Autodesk Inventor part; units mm, degrees
ref_plane "YZ Plane" through (0, 0, 0) normal (1, 0, 0) x (0, 1, 0)
ref_plane "XZ Plane" through (0, 0, 0) normal (0, 1, 0) x (-1, 0, 0)
ref_plane "XY Plane" through (0, 0, 0) normal (0, 0, 1) x (1, 0, 0)
sketch "スケッチ1" plane through (0, 0, 0) normal (0, 0, 1) x (1, 0, 0)
  line L0 (-40, 18) -> (40, 18)
  line L1 (40, 18) -> (40, -18)
  line L2 (40, -18) -> (-40, -18)
  line L3 (-40, -18) -> (-40, 18)
  line L4 (0, 0) -> (0, 18) construction
  line L5 (0, 0) -> (40, 0) construction
  dimension "d0" = 36
  dimension "d1" = 80
extrude "プレート1" add sketch "スケッチ1" along normal blind 5
sketch "スケッチ2" plane through (0, 0, 5) normal (0, 0, 1) x (1, 0, 0)
  line L0 (40, 18) -> (40, -18)
  line L1 (-40, 18) -> (-40, -18)
  line L2 (-40, 0) -> (40, 0) construction
  point P0 (22, 0)
  point P1 (11.8, 0)
  point P2 (27.1, -8.8335)
  point P3 (27.1, 8.8335)
  dimension "d3" = 10.2
  dimension "d6" = 360
  dimension "d116" = 18
hole "穴1" at (11.8, 0, 5) at (27.1, -8.8335, 5) at (27.1, 8.8335, 5) direction (0, 0, -1) diameter 4 depth 5
sketch "スケッチ3" plane through (0, 0, 5) normal (0, 0, 1) x (1, 0, 0)
  line L0 (40, 18) -> (40, -18)
  point P0 (22, 0)
  point P1 (22, -12.5)
  point P2 (32.8253, -6.25)
  point P3 (32.8253, 6.25)
  point P4 (22, 12.5)
  point P5 (11.1747, 6.25)
  point P6 (11.1747, -6.25)
  dimension "d15" = 12.5
  dimension "d18" = 360
  dimension "d117" = 18
hole "穴2" at (22, -12.5, 5) at (32.8253, -6.25, 5) at (32.8253, 6.25, 5) at (22, 12.5, 5) at (11.1747, 6.25, 5) at (11.1747, -6.25, 5) direction (0, 0, -1) diameter 3.2 depth 5
sketch "スケッチ13" plane through (0, 0, 0) normal (0, 0, -1) x (-1, 0, 0)
  line L0 (0, 0) -> (40, 0) construction
  line L1 (40, -18) -> (40, 18)
  line L2 (-40, 18) -> (-40, -18)
  point P0 (33, 0)
  point P1 (3, 0)
  dimension "d127" = 30
  dimension "d128" = 43
hole "穴10" at (-33, 0, 0) at (-3, 0, 0) direction (0, 0, 1) diameter 7.9 depth 5
fillet "フィレット1" radius 10 4 edges at (40, -18, 2.5) (40, 18, 2.5) (-40, 18, 2.5) (-40, -18, 2.5)
equation "\"d13\" = d3"
equation "\"d125\" = Thickness"
equation "\"d2\" = Thickness"
equation "\"BendRadius\" = Thickness"
equation "\"BendReliefWidth\" = Thickness"
equation "\"BendReliefDepth\" = 0.5 * Thickness"
equation "\"TransitionRadius\" = BendRadius"
equation "\"JacobiRadiusSize\" = BendRadius"
equation "\"GapSize\" = Thickness"
properties part number "link_plate" material "アルミニウム 6061"
CAD build for the part. Positions are in the model's coordinates, mm. Round coordinates to 2 decimals unless told otherwise and drop trailing zeros. Loops run counter-clockwise (first coordinate to the right, second up) from the corner with the lowest first, then second, coordinate; pieces in that order, holes last. Notation, with made-up numbers: M -1,23.5 L 25,23.5 A35 ccw 25,60.5 Z; hole C -2.5,54 d5. An arc over 180 degrees is marked long. Use a Markdown table: item, result. Add a question column.
(1) Cut at B-B (y = 0). Give the cut face in (x, z).
(2) Flat gauge pins, fed straight in: pin 1 (3 mm diameter, centred on y = -11.5, z = 1, fed in from +X); pin 2 (2.5 mm diameter, centred on x = 22, y = 12.5, fed in from +Z); pin 3 (1 mm diameter, centred on y = 14, z = 2.5, fed in from -X). Where does each tip first touch, or does it go through?
(3) Cut at D-D (z = 3.7). State how many separate pieces and enclosed holes the cut face has, and give its area (3 significant figures).
(4) Cut at C-C (y = -12.5). Give the cut face in (x, z), and give its area (3 significant figures).
(5) Cut at A-A (x = 22). Give the cut face in (y, z), and give its area (3 significant figures).
(6) Pull direction X, two halves, no side cores. Call faces 1 (the face through (9.817, 0.26, 2.465)), 2 (the face through (-40, 0, 2)), 3 (the face through (0, 18, 2)): +X half, -X half, draft (parallel to the pull), parting line (faces both ways), or undercut.
(7) Drill centre lines: line 1 (X direction, y = 0, z = 2.25); line 2 (X direction, y = 6.25, z = 2.4); line 3 (Y direction, x = 22.5, z = 1.75). Where is each one in solid material? Low to high.
Geometry says:
| question | item | result |
|---|---|---|
| 1 | outline | M -40,0 L -36.95,0 L -36.95,5 L -40,5 Z; M -29.05,0 L -6.95,0 L -6.95,5 L -29.05,5 Z; M 0.95,0 L 9.8,0 L 9.8,5 L 0.95,5 Z; M 13.8,0 L 40,0 L 40,5 L 13.8,5 Z |
| 2 | pin 1 | stops at x = 39.8 |
| 2 | pin 2 | passes through |
| 2 | pin 3 | stops at x = -38.35 |
| 3 | separate pieces | 1 |
| 3 | enclosed holes | 11 |
| 3 | area | 2,610 mm² |
| 4 | outline | M -38.93,0 L 20.4,0 L 20.4,5 L -38.93,5 Z; M 23.6,0 L 38.93,0 L 38.93,5 L 23.6,5 Z |
| 4 | area | 373 mm² |
| 5 | outline | M -18,0 L -14.1,0 L -14.1,5 L -18,5 Z; M -10.9,0 L 10.9,0 L 10.9,5 L -10.9,5 Z; M 14.1,0 L 18,0 L 18,5 L 14.1,5 Z |
| 5 | area | 148 mm² |
| 6 | face 1 | undercut |
| 6 | face 2 | -X half |
| 6 | face 3 | draft |
| 7 | line 1 | x = -40 to -36.95, -29.05 to -6.95, 0.95 to 9.8, 13.8 to 40 |
| 7 | line 2 | x = -40 to 9.57, 12.77 to 31.23, 34.43 to 40 |
| 7 | line 3 | y = -18 to -14.02, -10.98 to 10.98, 14.02 to 18 |
